Geometry: final body of the model. Coordinates: model frame, mm. Face numbers are marked on the shaded views. A direction names the side the tool comes from. Give positions to 0.01 mm unless a question says otherwise; leave off trailing zeros. Order: outer loops, then holes, each group sorted by start corner. A loop starts at its lowest first (then second) coordinate and runs counter-clockwise, first axis right, second up. Notation, with made-up numbers: (65.25, 9) - (90.25, 9) arc R33 ccw to (90.25, 39) - close; hole circle Ø10 at (46, 12). An arc over 180 degrees is marked (long way). Put each result on its own line as item: value. Start each with the question number.
1. First-contact query: P1, Ø10, axis at x = -11.5, y = -12.5, coming from the +Z side; P2, Ø10, axis at x = -36.5, y = -32, coming from the -Z side; P3, Ø8, axis at x = -78, z = 71.5, coming from the -Y side. Flat tips, straight axial feed; report the tip coordinate or a pass-through.
2. Ray query, line 1 along Y through (x, z) = (-92, 90.5); line 2 along X through (y, z) = (-29.5, 67); line 3 along Z through (x, y) = (-9.5, -23). Return the intervals inside material, ascending. Write a range as from..to.
3. Mould query, pull axis Y, two halves, no side actions, for the marked faces 3, 4 and 5. Classes: pulls with the +Y half, pulls with the -Y half, needs draft (parallel to the pull), parting line crosses it, or undercut.
4. Section B-B on x = -61. Return the cut outline in (y, z), plus the area to 3 significant figures.
5. Set-up query: the marked faces 1 and 2. Return all of +Z, -Z, +X, -X, +Y, -Y with unobstructed straight access to the full face (end or side cutting, diameter ignored); none if empty.
6. Section C-C on z = 37.5. Return the cut outline in (x, y), plus the area to 3 significant figures.
7. Section D-D on y = -25. Return the cut outline in (x, z).
8. Section A-A on x = -32. Return the cut outline in (y, z), plus the area to 3 significant figures.
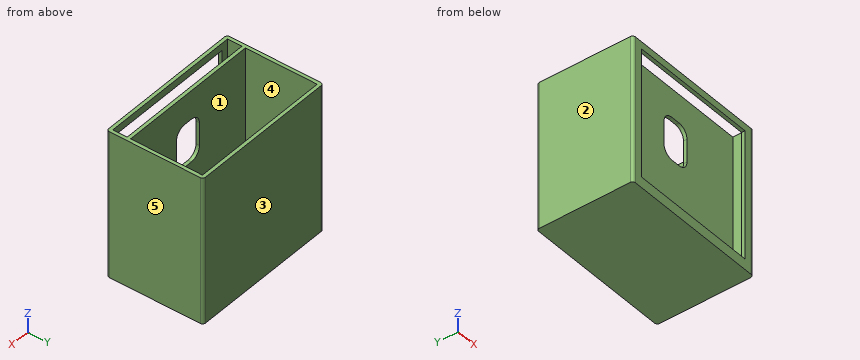
from build123d import *

# Parameters (mm, degrees)
SKETCH_W        = 104.8
SKETCH_H        = 102.4
PAD_DEPTH       = 67.2
SKETCH001_W     = 100
SKETCH001_H     = 50
POCKET_DEPTH    = 100
SKETCH002_W     = 100
SKETCH002_H     = 10
POCKET001_DEPTH = 100
SKETCH003_W     = 90
SKETCH003_H     = 90
POCKET002_DEPTH = 3
SKETCH004_W     = 20
SKETCH004_H     = 30
POCKET003_DEPTH = 5
FILLET_R        = 2
FILLET001_R     = 2
FILLET002_R     = 2
FILLET003_R     = 2
FILLET004_R     = 7
FILLET005_R     = 7
FILLET006_R     = 7
FILLET007_R     = 7


with BuildPart() as part:
    # Sketch → Pad (new body)
    with BuildSketch(Plane.XZ):
        with Locations((-52.4, 51.2)):
            Rectangle(SKETCH_W, SKETCH_H)
    extrude(amount=PAD_DEPTH)

    # Sketch001 (on Face1 of Pad) → Pocket (cut)
    with BuildSketch(Plane(origin=(0, 0, 102.4), x_dir=(-1, 0, 0), z_dir=(0, 0, 1))):
        with Locations((52.4, 27.4)):
            Rectangle(SKETCH001_W, SKETCH001_H)
    extrude(amount=-POCKET_DEPTH, mode=Mode.SUBTRACT)

    # Sketch002 (on Face1 of Pocket) → Pocket001 (cut)
    with BuildSketch(Plane(origin=(0, 0, 102.4), x_dir=(-1, 0, 0), z_dir=(0, 0, 1))):
        with Locations((52.4, 59.8)):
            Rectangle(SKETCH002_W, SKETCH002_H)
    extrude(amount=-POCKET001_DEPTH, mode=Mode.SUBTRACT)

    # Sketch003 (on Face4 of Pocket001) → Pocket002 (cut)
    with BuildSketch(Plane.XZ.offset(67.2)):
        with Locations((-52.4, 52.4)):
            Rectangle(SKETCH003_W, SKETCH003_H)
    extrude(amount=-POCKET002_DEPTH, mode=Mode.SUBTRACT)

    # Sketch004 (on Face7 of Pocket002) → Pocket003 (cut)
    with BuildSketch(Plane.XZ.offset(54.8)):
        with Locations((-52.4, 67.4)):
            Rectangle(SKETCH004_W, SKETCH004_H)
    extrude(amount=-POCKET003_DEPTH, mode=Mode.SUBTRACT)

    # Fillet
    fillet_edges = [part.edges().sort_by_distance(p)[0] for p in [
        (0, -67.2, 51.2),
    ]]
    fillet(fillet_edges, radius=FILLET_R)

    # Fillet001
    fillet001_edges = [part.edges().sort_by_distance(p)[0] for p in [
        (-104.8, -67.2, 51.2),
    ]]
    fillet(fillet001_edges, radius=FILLET001_R)

    # Fillet002
    fillet002_edges = [part.edges().sort_by_distance(p)[0] for p in [
        (-104.8, 0, 51.2),
    ]]
    fillet(fillet002_edges, radius=FILLET002_R)

    # Fillet003
    fillet003_edges = [part.edges().sort_by_distance(p)[0] for p in [
        (0, 0, 51.2),
    ]]
    fillet(fillet003_edges, radius=FILLET003_R)

    # Fillet004
    fillet004_edges = [part.edges().sort_by_distance(p)[0] for p in [
        (-62.4, -53.6, 52.4),
    ]]
    fillet(fillet004_edges, radius=FILLET004_R)

    # Fillet005
    fillet005_edges = [part.edges().sort_by_distance(p)[0] for p in [
        (-42.4, -53.6, 52.4),
    ]]
    fillet(fillet005_edges, radius=FILLET005_R)

    # Fillet006
    fillet006_edges = [part.edges().sort_by_distance(p)[0] for p in [
        (-42.4, -53.6, 82.4),
    ]]
    fillet(fillet006_edges, radius=FILLET006_R)

    # Fillet007
    fillet007_edges = [part.edges().sort_by_distance(p)[0] for p in [
        (-62.4, -53.6, 82.4),
    ]]
    fillet(fillet007_edges, radius=FILLET007_R)


solid = part.part
Resolved:
1. P1: z = 2.4
1. P2: z = 0
1. P3: y = -54.8
2. line 1: -54.8..-52.4, -2.4..0
2. line 2: -104.8..-102.4, -2.4..0
2. line 3: 0..2.4
3. face 3: pulls with the +Y half
3. face 4: undercut
3. face 5: needs draft
4. outline: (-67.2, 0) - (0, 0) - (0, 102.4) - (-2.4, 102.4) - (-2.4, 2.4) - (-52.4, 2.4) - (-52.4, 55.2) - (-54.8, 55.2) - (-54.8, 2.4) - (-64.8, 2.4) - (-64.8, 7.4) - (-67.2, 7.4) - close; (-67.2, 97.4) - (-64.8, 97.4) - (-64.8, 102.4) - (-67.2, 102.4) - close; (-54.8, 79.6) - (-52.4, 79.6) - (-52.4, 102.4) - (-54.8, 102.4) - close
4. area: 607 mm^2
5. face 1: +Z
5. face 2: +Z, -Z, -X, +Y, -Y
6. outline: (-104.8, -65.2) arc R2 ccw to (-102.8, -67.2) - (-97.4, -67.2) - (-97.4, -64.8) - (-102.4, -64.8) - (-102.4, -54.8) - (-2.4, -54.8) - (-2.4, -64.8) - (-7.4, -64.8) - (-7.4, -67.2) - (-2, -67.2) arc R2 ccw to (0, -65.2) - (0, -2) arc R2 ccw to (-2, 0) - (-102.8, 0) arc R2 ccw to (-104.8, -2) - close; hole (-102.4, -52.4) - (-2.4, -52.4) - (-2.4, -2.4) - (-102.4, -2.4) - close
6. area: 823 mm^2
7. outline: (-104.8, 0) - (0, 0) - (0, 102.4) - (-2.4, 102.4) - (-2.4, 2.4) - (-102.4, 2.4) - (-102.4, 102.4) - (-104.8, 102.4) - close
8. outline: (-67.2, 0) - (0, 0) - (0, 102.4) - (-2.4, 102.4) - (-2.4, 2.4) - (-52.4, 2.4) - (-52.4, 102.4) - (-54.8, 102.4) - (-54.8, 2.4) - (-64.8, 2.4) - (-64.8, 7.4) - (-67.2, 7.4) - close; (-67.2, 97.4) - (-64.8, 97.4) - (-64.8, 102.4) - (-67.2, 102.4) - close
8. area: 665 mm^2
